Job drawing, mm, ordinate dimensions from the low corner. One solid piece. A direction names the side the tool comes from. Round coordinates to 2 decimals unless told otherwise and drop trailing zeros. Write each loop counter-clockwise with the first axis right and the second up, starting at its lowest first coordinate (ties: lowest second). Pieces come first, ordered by that corner, then holes. Notation, with made-up numbers: M 31.5,-5.5 L 69.5,-5.5 A11 ccw 69.5,10.5 Z; hole C 7,37.25 d1. An arc over 180 degrees is marked long. Answer as a JSON object with one key per item and string values. Group by question number.
1. Band-saw the part on A-A, the plane y = 52. Write the cut outline in (x, z), plus the area to 3 significant figures.
2. Drill centre lines: line 1 (Y direction, x = 27, z = 0.85); line 2 (Z direction, x = 1.4, y = 52); line 3 (X direction, y = 23.5, z = 4.5). Where is each one in solid material? Low to high. Write a range as from..to.
3. Drop flat-ended pins along their axis: pin 1 (6 mm diameter, centred on x = 8.5, y = 68.5, fed in from +Z); pin 2 (2.5 mm diameter, centred on x = 27, y = 72, fed in from -Z). Give the stop position or say it passes through.
4. Band-saw the part on B-B, the plane x = 27. Write the cut outline in (y, z).
5. Which spindle directions (+Z, -Z, +X, -X, +Y, -Y) get a long thin tool onto all of the face, cutting with end or side? Do the marked faces 1 and 2. Say none if no direction does.
6. Band-saw the part on C-C, the plane z = 6.2. Write the cut outline in (x, y), plus the area to 3 significant figures.
7. Band-saw the part on D-D, the plane y = 37. Write the cut outline in (x, z).
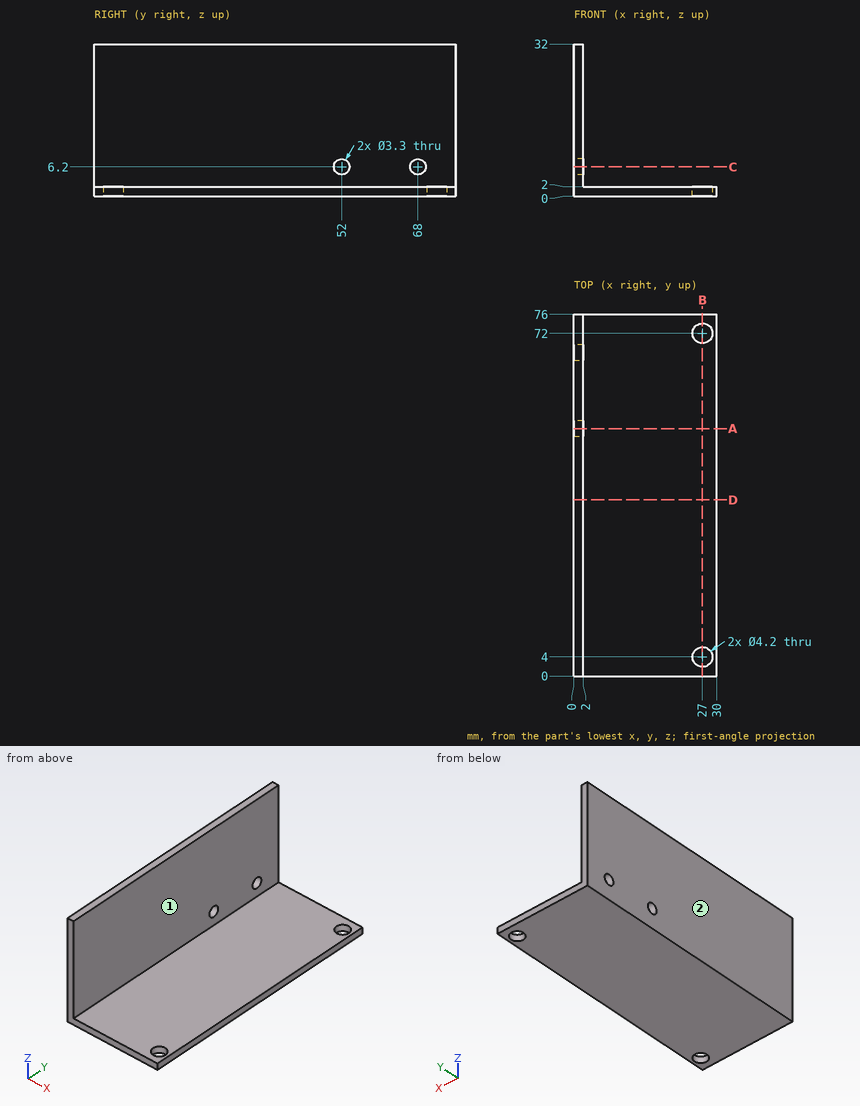
Worked answers:
{
 "1": {"outline": "M 0,0 L 30,0 L 30,2 L 2,2 L 2,4.55 L 0,4.55 Z; M 0,7.85 L 2,7.85 L 2,32 L 0,32 Z", "area": "113 mm^2"},
 "2": {"line 1": "y = 0..1.9, 6.1..69.9, 74.1..76", "line 2": "z = 0..4.55, 7.85..32", "line 3": "x = 0..2"},
 "3": {"pin 1": "stops at z = 2", "pin 2": "passes through"},
 "4": {"outline": "M 0,0 L 1.9,0 L 1.9,2 L 0,2 Z; M 6.1,0 L 69.9,0 L 69.9,2 L 6.1,2 Z; M 74.1,0 L 76,0 L 76,2 L 74.1,2 Z"},
 "5": {"face 1": "+Z, +X, +Y, -Y", "face 2": "+Z, -Z, -X, +Y, -Y"},
 "6": {"outline": "M 0,0 L 2,0 L 2,50.35 L 0,50.35 Z; M 0,53.65 L 2,53.65 L 2,66.35 L 0,66.35 Z; M 0,69.65 L 2,69.65 L 2,76 L 0,76 Z", "area": "139 mm^2"},
 "7": {"outline": "M 0,0 L 30,0 L 30,2 L 2,2 L 2,32 L 0,32 Z"}
}
